Job drawing, mm, ordinate dimensions from the low corner. One solid piece. A direction names the side the tool comes from. Give positions to 0.01 mm unless a question says otherwise; leave off trailing zeros. Write each loop counter-clockwise with the first axis right and the second up, starting at its lowest first coordinate (ties: lowest second). Pieces come first, ordered by that corner, then holes. Notation, with made-up numbers: (73.5, -29.5) - (102.5, -29.5) arc R10 ccw to (102.5, -23.5) - close; hole circle Ø4 at (50, 27.25). An arc over 180 degrees is marked (long way). Answer as a JSON object with one key per item and string values.
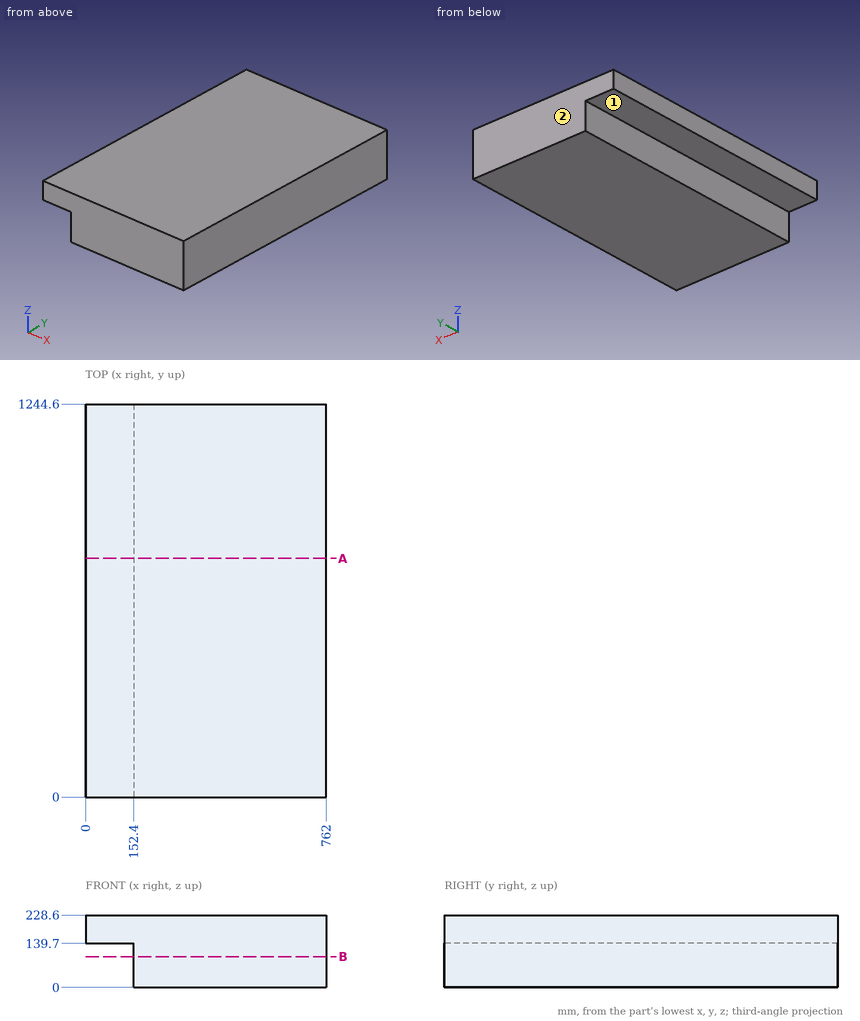
Item 1: Cut at B-B (z = 97.5). Give the cut face in (x, y), and give its area (3 significant figures).
Entries:
{"outline": "(152.4, 0) - (762, 0) - (762, 1244.6) - (152.4, 1244.6) - close", "area": "759,000 mm2"}
Item 2: Probe line 1 (X direction, y = 109, z = 51.5); line 2 (Z direction, x = 98.5, y = 942). List the from-to ranges inside material, lowest first. Write a range as from..to.
Entries:
{"line 1": "152.4..762", "line 2": "139.7..228.6"}
Item 3: Which spindle directions (+Z, -Z, +X, -X, +Y, -Y) get a long thin tool onto all of the face, cutting with end or side? Do the marked faces 1 and 2. Say none if no direction does.
Entries:
{"face 1": "-Z, -X, +Y, -Y", "face 2": "+Z, -Z, +X, -X, +Y"}
Item 4: Flat gauge pin, fed straight in: P1, Ø3, axis at y = 221.5, z = 104, coming from the -X side. Where does the tip first touch, or does it go through?
Entries:
{"P1": "x = 152.4"}
Item 5: Cut at A-A (y = 756). Give the cut face in (x, z).
Entries:
{"outline": "(0, 139.7) - (152.4, 139.7) - (152.4, 0) - (762, 0) - (762, 228.6) - (0, 228.6) - close"}
